```python
from build123d import *

# Parameters (mm, degrees)
SKETCH1_R           = 1.65
BOSS_EXTRUDE2_DEPTH = 3.175


with BuildPart() as part:
    # Sketch1 → Boss-Extrude2 (new body)
    with BuildSketch(Plane(origin=(0, 0, 0), x_dir=(1, 0, 0), z_dir=(0, 1, 0))):
        with BuildLine():
            Line((-55.306734792, 42.908799641), (-55.306734792, 22.908799641))
            Line((-55.306734792, 22.908799641), (55.306734792, 22.908799641))
            Line((55.306734792, 22.908799641), (55.306734792, 42.908799641))
            ThreePointArc((55.306734792, 42.908799641), (0, 70), (-55.306734792, 42.908799641))
        make_face()
        with Locations((35, 48.621778265)):
            Circle(SKETCH1_R, mode=Mode.SUBTRACT)
        with Locations((35, 30.621778265)):
            Circle(SKETCH1_R, mode=Mode.SUBTRACT)
        with Locations((-35, 30.621778265)):
            Circle(SKETCH1_R, mode=Mode.SUBTRACT)
        with Locations((-35, 48.621778265)):
            Circle(SKETCH1_R, mode=Mode.SUBTRACT)
    extrude(amount=BOSS_EXTRUDE2_DEPTH)


solid = part.part
```
Model file for the job. Use its own axes, mm. Round coordinates to 2 decimals unless told otherwise and drop trailing zeros. Write each loop counter-clockwise with the first axis right and the second up, starting at its lowest first coordinate (ties: lowest second). Pieces come first, ordered by that corner, then holes. Notation, with made-up numbers: (74.25, -4.5) - (87.25, -4.5) arc R19 ccw to (87.25, 25.5) - close; hole circle Ø11 at (-27, 8.25). An arc over 180 degrees is marked (long way). One line per item, written item: value.
(1) Cut at B-B, the plane x = -35. Give the cut face in (y, z) (3 decimals), plus the area to 3 significant figures.
Values follow:
outline: (0, -60.622) - (3.175, -60.622) - (3.175, -50.272) - (0, -50.272) - close; (0, -46.972) - (3.175, -46.972) - (3.175, -32.272) - (0, -32.272) - close; (0, -28.972) - (3.175, -28.972) - (3.175, -22.909) - (0, -22.909) - close
area: 98.8 mm²
(2) Drop a flat-ended pin along its axis: P1, Ø1.5, axis at y = 2, z = -62, coming from the -X side. Give the stop position or say it passes through.
Values follow:
P1: stops at x = -33.89
(3) Cut at D-D, the plane x = 48. Give the cut face in (y, z) (3 decimals), plus the area to 3 significant figures.
Values follow:
outline: (0, -50.951) - (3.175, -50.951) - (3.175, -22.909) - (0, -22.909) - close
area: 89.0 mm²
(4) Cut at A-A, the plane y = 1.3. Give the cut face in (x, z).
Values follow:
outline: (-55.31, -42.91) arc R70 ccw to (55.31, -42.91) - (55.31, -22.91) - (-55.31, -22.91) - close; hole circle Ø3.3 at (-35, -48.62); hole circle Ø3.3 at (-35, -30.62); hole circle Ø3.3 at (35, -48.62); hole circle Ø3.3 at (35, -30.62)
(5) Cut at C-C, the plane z = -59. Give the cut face in (x, y) (3 decimals).
Values follow:
outline: (-37.67, 0) - (37.67, 0) - (37.67, 3.175) - (-37.67, 3.175) - close
(6) Wall check: probe 1 along X at (y, z) = (1.3, -29.5); probe 2 along Z at (x, y) = (-35, 0.85); probe 3 along X at (y, z) = (2.9, -32). Give the ranges that are in metal, low to high.
Values follow:
probe 1: x = -55.31 to -36.21, -33.79 to 33.79, 36.21 to 55.31
probe 2: z = -60.62 to -50.27, -46.97 to -32.27, -28.97 to -22.91
probe 3: x = -55.31 to -35.91, -34.09 to 34.09, 35.91 to 55.31
(7) Two-plate mould, pull along Z, no slides. Class faces 1 (the flat face through (-1, 3.175, -42)), 2 (the cylindrical face through (0.893, 1.565, -69.994)), 3 (the cylindrical face through (-35.21, 1.57, -32.26)): pulls with the +Z half, pulls with the -Z half, needs draft (parallel to the pull), parting line crosses it, or undercut.
Values follow:
face 1: needs draft
face 2: pulls with the -Z half
face 3: undercut
